Autodesk Inventor part; units mm, degrees
ref_plane "Arbeitsebene1" through (0, -0.5, 0) normal (0, 1, 0) x (1, 0, 0)
ref_plane "YZ Plane" through (0, 0, 0) normal (1, 0, 0) x (0, 1, 0)
ref_plane "XZ Plane" through (0, 0, 0) normal (0, 1, 0) x (-1, 0, 0)
sketch "Skizze1" plane through (0, 0, 0) normal (0, 1, 0) x (-1, 0, 0)
  circle A0 centre (0, 0) radius 3.5
  line L0 (5.875, -5.875) -> (-5.875, -5.875)
  line L1 (-5.875, -5.875) -> (-5.875, 5.875)
  line L2 (-5.875, 5.875) -> (5.875, 5.875)
  line L3 (5.875, 5.875) -> (5.875, -5.875)
  line L4 (8.225, 0) -> (-8.225, 0)
  line L5 (0.75, 5.875) -> (-0.75, 5.875)
  line L6 (0, -8.225) -> (0, 8.225)
  point P0 (0.75, -5.875)
  point P1 (-5.875, -0.75)
  point P2 (5.875, -0.75)
  dimension "d1" = 7
  dimension "d2" = 11.75
  dimension "d3" = 11.75
extrude "Extrusion1" add sketch "Skizze1" along normal mid plane 6
sketch "Skizze2" plane through (0, 3, 0) normal (0, 1, 0) x (1, 0, 0)
  circle A0 centre (0, 0) radius 3
  dimension "d14" = 6
ref_plane "Arbeitsebene1" through (0, -0.5, 0) normal (0, 1, 0) x (1, 0, 0)
sketch "Skizze4" plane through (0, -3, 0) normal (0, -1, 0) x (1, 0, 0)
  circle A0 centre (0, 0) radius 2.85
  circle A1 centre (0, 0) radius 1.4
  circle A2 centre (0, 0) radius 4.1
  dimension "d20" = 5.7
  dimension "d21" = 8.2
extrude "Extrusion4" add sketch "Skizze4" along normal blind 2.5 contours A2
sketch "Skizze5" plane through (0, 3, 0) normal (0, 1, 0) x (1, 0, 0)
  line L0 (-5.875, 5.875) -> (5.875, 5.875)
  line L1 (-5.875, 5.875) -> (-3.775, 5.875)
  line L2 (-3.775, 5.875) -> (-3.775, 3.775)
  line L3 (-3.775, 3.775) -> (-5.875, 3.775)
  line L4 (-5.875, 3.775) -> (-5.875, 5.875)
  line L5 (-5.875, 5.875) -> (5.875, 5.875)
  line L6 (5.875, 5.875) -> (3.775, 5.875)
  line L7 (3.775, 5.875) -> (3.775, 3.775)
  line L8 (3.775, 3.775) -> (5.875, 3.775)
  line L9 (5.875, 3.775) -> (5.875, 5.875)
  line L10 (-5.875, -5.875) -> (-5.875, 5.875)
  line L11 (-5.875, -5.875) -> (-3.775, -5.875)
  line L12 (-3.775, -5.875) -> (-3.775, -3.775)
  line L13 (-3.775, -3.775) -> (-5.875, -3.775)
  line L14 (-5.875, -3.775) -> (-5.875, -5.875)
  line L15 (5.875, -5.875) -> (-5.875, -5.875)
  line L16 (5.875, -5.875) -> (3.775, -5.875)
  line L17 (3.775, -5.875) -> (3.775, -3.775)
  line L18 (3.775, -3.775) -> (5.875, -3.775)
  line L19 (5.875, -3.775) -> (5.875, -5.875)
  point P0 (0, 0)
  point P1 (-0.75, 5.75)
  point P2 (0.75, 5.75)
  point P3 (-5.75, -0.75)
  point P4 (0.75, -5.75)
  dimension "d24" = 2.1
  dimension "d25" = 2.1
  dimension "d26" = 2.1
  dimension "d27" = 2.1
  dimension "d28" = 2.1
  dimension "d29" = 2.1
  dimension "d30" = 2.1
  dimension "d31" = 2.1
extrude "Extrusion5" cut sketch "Skizze5" against normal blind 6
extrude "Extrusion6" cut sketch "Skizze2" against normal blind 1
sketch "Skizze6" plane through (0, 2, 0) normal (0, 1, 0) x (1, 0, 0)
  circle A0 centre (0, 0) radius 1.5
  dimension "d38" = 3
extrude "Extrusion7" cut sketch "Skizze6" against normal up to surface (5 mm away)
properties part number "_3D-Druck"
CAD build for the part. Positions are in the model's coordinates, mm. A direction names the side the tool comes from. Coordinates: 2 decimals unless noted, no trailing zeros. Loops run counter-clockwise (first coordinate to the right, second up) from the corner with the lowest first, then second, coordinate; pieces in that order, holes last. Notation, with made-up numbers: (27, 77) - (50, 77) arc R33 ccw to (50, 116) - close; hole circle Ø3 at (29, 52.5). An arc over 180 degrees is marked (long way). Write item = value, one per line. Start each with the question number.
Q1. Flat gauge pins, fed straight in: pin 1 Ø4.5 at (x, z) = (0, 0) entering from -Y; pin 2 Ø0.6 at (x, y) = (-5, 0) entering from +Z (3 decimals); pin 3 Ø5.5 at (x, z) = (0, 0) entering from +Y. Where does each tip first touch, or does it go through?
Q2. Cut at B-B, the plane z = 0. List the corners of the cut face in (x, y) (3 decimals), then the cut area to 4 significant figures.
Q3. Cut at C-C, the plane x = 0. List the corners of the cut face in (y, z) (3 decimals).
Q4. Cut at D-D, the plane z = -2. List the corners of the cut face in (x, y) (3 decimals), then the cut area to 3 significant figures.
Q5. Which spindle directions (+Z, -Z, +X, -X, +Y, -Y) get a long thin tool onto all of the face, cutting with end or side? Do faces 5 (the flat face through (3.775, 0, -5)), 6 (the flat face through (1.3, 2, 1.3)), 7 (the flat face through (-5, 0, 3.775)), 8 (the flat face through (-3.775, 0, -5)), 9 (the cylindrical face through (-0.534, -4.232, -4.065)). Say none if no direction does.
Q6. Cut at A-A, the plane y = -0.75. List the corners of the cut face in (x, z) (3 decimals).
Q7. Drill centre lines: L1, parallel to Z at x = 0, y = -0.3 (3 decimals); L2, parallel to Z at x = 0, y = -4.75; L3, parallel to X at y = 2.55, z = 0 (3 decimals). Where is each one in solid material? Low to high.
Q8. Pull direction Z, two halves, no side cores. Call faces 1 (the flat face through (-1.2, -3, -1.2)), 2 (the flat face through (-5, 0, -3.775)), 3 (the cylindrical face through (-2.262, -4.232, 1.734)), 4 (the flat face through (3, -3, 4)): pulls with the +Z half, pulls with the -Z half, needs draft (parallel to the pull), parting line crosses it, or undercut.
Computed:
q1.pin_1 = -3
q1.pin_2 = 3.775
q1.pin_3 = 2
q2.outline = (-5.875, -3) - (-4.1, -3) - (-4.1, -5.5) - (-2.85, -5.5) - (-2.85, -3) - (-1.5, -3) - (-1.5, 2) - (-3, 2) - (-3, 3) - (-5.875, 3) - close; (1.5, -3) - (2.85, -3) - (2.85, -5.5) - (4.1, -5.5) - (4.1, -3) - (5.875, -3) - (5.875, 3) - (3, 3) - (3, 2) - (1.5, 2) - close
q2.area = 55.75 mm²
q3.outline = (-5.5, -4.1) - (-3, -4.1) - (-3, -5.875) - (3, -5.875) - (3, -3) - (2, -3) - (2, -1.5) - (-3, -1.5) - (-3, -2.85) - (-5.5, -2.85) - close; (-5.5, 2.85) - (-3, 2.85) - (-3, 1.5) - (2, 1.5) - (2, 3) - (3, 3) - (3, 5.875) - (-3, 5.875) - (-3, 4.1) - (-5.5, 4.1) - close
q4.outline = (-5.875, -3) - (-3.579, -3) - (-3.579, -5.5) - (-2.03, -5.5) - (-2.03, -3) - (2.03, -3) - (2.03, -5.5) - (3.579, -5.5) - (3.579, -3) - (5.875, -3) - (5.875, 3) - (2.236, 3) - (2.236, 2) - (-2.236, 2) - (-2.236, 3) - (-5.875, 3) - close
q4.area = 73.8 mm²
q5.face_5 = -Z, +X, +Y, -Y
q5.face_6 = +Y
q5.face_7 = +Z, -X, +Y, -Y
q5.face_8 = -Z, -X, +Y, -Y
q5.face_9 = -Y
q6.outline = (-5.875, -3.775) - (-3.775, -3.775) - (-3.775, -5.875) - (3.775, -5.875) - (3.775, -3.775) - (5.875, -3.775) - (5.875, 3.775) - (3.775, 3.775) - (3.775, 5.875) - (-3.775, 5.875) - (-3.775, 3.775) - (-5.875, 3.775) - close; hole circle Ø3 at (0, 0)
q7.L1 = -5.875 to -1.5, 1.5 to 5.875
q7.L2 = -4.1 to -2.85, 2.85 to 4.1
q7.L3 = -5.875 to -3, 3 to 5.875
q8.face_1 = undercut
q8.face_2 = pulls with the -Z half
q8.face_3 = undercut
q8.face_4 = needs draft
